```python
from build123d import *

# Parameters (mm, degrees)
SKETCH11_RX                  = 55.88
SKETCH11_RY                  = 50.8
BOSS_EXTRUDE4_DEPTH          = 9.525
SKETCH14_R                   = 0.0001
CUT_EXTRUDE5_DEPTH           = 10.525
CUT_EXTRUDE4_DEPTH           = 10.525
LPATTERN1_COUNT              = 4
LPATTERN1_PITCH              = 3.5
LPATTERN1_COL_COUNT          = 4
LPATTERN1_COL_PITCH          = 3.5
MIRROR1_COPY_1_DEPTH         = 10.525
MIRROR1_COPY_2_DEPTH         = 10.525
MIRROR1_COPY_3_DEPTH         = 10.525
MIRROR1_COPY_4_DEPTH         = 10.525
MIRROR1_COPY_5_DEPTH         = 10.525
MIRROR1_COPY_6_DEPTH         = 10.525
F_1_8_0_125_DIAMETER_HOLE1_D = 3.175


with BuildPart() as part:
    # Sketch11 → Boss-Extrude4 (new body)
    with BuildSketch(Plane(origin=(0, 0, 0), x_dir=(1, 0, 0), z_dir=(0, 1, 0))):
        with Locations(Location((0, 0), (0, 0, 180))):
            Ellipse(SKETCH11_RX, SKETCH11_RY)
        with BuildLine():
            Line((-32.5125, 22.448135593), (32.5125, 22.448135593))
            ThreePointArc((32.5125, 22.448135593), (40.370224106, 19.193359699), (43.625, 11.335635593))
            Line((43.625, 11.335635593), (43.625, -11.335635593))
            ThreePointArc((43.625, -11.335635593), (40.370224106, -19.193359699), (32.5125, -22.448135593))
            Line((32.5125, -22.448135593), (-32.5125, -22.448135593))
            ThreePointArc((-32.5125, -22.448135593), (-40.370224106, -19.193359699), (-43.625, -11.335635593))
            Line((-43.625, -11.335635593), (-43.625, 11.335635593))
            ThreePointArc((-43.625, 11.335635593), (-40.370224106, 19.193359699), (-32.5125, 22.448135593))
        make_face(mode=Mode.SUBTRACT)
    extrude(amount=BOSS_EXTRUDE4_DEPTH)

    # Sketch14 → Cut-Extrude5 (cut, through all)
    with BuildSketch(Plane(origin=(0, 9.525, 0), x_dir=(1, 0, 0), z_dir=(0, 1, 0))):
        with Locations((-25.4, 28.798235593)):
            Circle(SKETCH14_R)
        with Locations((25.4, 28.798235593)):
            Circle(SKETCH14_R)
        with Locations((25.4, 38.323035593)):
            Circle(SKETCH14_R)
        with Locations((-25.4, 38.323035593)):
            Circle(SKETCH14_R)
        with BuildLine():
            Line((-25.4, 38.323135593), (-6.981368472, 38.323135593))
            ThreePointArc((-6.981368472, 38.323135593), (-5.858836457, 38.788103578), (-5.393868472, 39.910635593))
            Line((-5.393868472, 39.910635593), (-5.393868472, 41.815635593))
            ThreePointArc((-5.393868472, 41.815635593), (-4.928900487, 42.938167608), (-3.806368472, 43.403135593))
            Line((-3.806368472, 43.403135593), (3.806368472, 43.403135593))
            ThreePointArc((3.806368472, 43.403135593), (4.928900487, 42.938167608), (5.393868472, 41.815635593))
            Line((5.393868472, 41.815635593), (5.393868472, 39.910635593))
            ThreePointArc((5.393868472, 39.910635593), (5.858836457, 38.788103578), (6.981368472, 38.323135593))
            Line((6.981368472, 38.323135593), (25.4001, 38.323035593))
            Line((25.4001, 38.323035593), (25.4, 28.798135593))
            Line((25.4, 28.798135593), (-25.4001, 28.798235593))
            Line((-25.4001, 28.798235593), (-25.4, 38.323135593))
        make_face()
    cut_extrude5 = extrude(amount=-CUT_EXTRUDE5_DEPTH, mode=Mode.SUBTRACT)

    # Sketch12 → Cut-Extrude4 (cut, through all)
    with BuildSketch(Plane(origin=(0, 9.525, 0), x_dir=(1, 0, 0), z_dir=(0, 1, 0))):
        with BuildLine():
            Line((-43.625, 0.81), (-47.625, 0.81))
            ThreePointArc((-47.625, 0.81), (-48.435, 0), (-47.625, -0.81))
            Line((-47.625, -0.81), (-43.625, -0.81))
            Line((-43.625, -0.81), (-43.625, 0.81))
        make_face()
    cut_extrude4 = extrude(amount=-CUT_EXTRUDE4_DEPTH, mode=Mode.SUBTRACT)

    # LPattern1: Cut-Extrude4 ×4
    with Locations(*[(0, 0, -i * LPATTERN1_PITCH) for i in range(1, LPATTERN1_COUNT)]):
        add(cut_extrude4, mode=Mode.SUBTRACT)

    # LPattern1 col: Cut-Extrude4 ×4
    with Locations(*[(0, 0, i * LPATTERN1_COL_PITCH) for i in range(1, LPATTERN1_COL_COUNT)]):
        add(cut_extrude4, mode=Mode.SUBTRACT)

    # Mirror1: Cut-Extrude4 across plane
    add(cut_extrude4.mirror(Plane(origin=(0, 0, 0), x_dir=(0, 0, 1), z_dir=(1, 0, 0))), mode=Mode.SUBTRACT)

    # Mirror1 copy 1 sketch → Mirror1 copy 1 (cut, through all)
    with BuildSketch(Plane(origin=(0, 9.525, -3.5), x_dir=(-1, 0, 0), z_dir=(0, 1, 0))):
        with BuildLine():
            Line((-43.625, -0.81), (-47.625, -0.81))
            ThreePointArc((-47.625, -0.81), (-48.435, 0), (-47.625, 0.81))
            Line((-47.625, 0.81), (-43.625, 0.81))
            Line((-43.625, 0.81), (-43.625, -0.81))
        make_face()
    extrude(amount=-MIRROR1_COPY_1_DEPTH, mode=Mode.SUBTRACT)

    # Mirror1 copy 2 sketch → Mirror1 copy 2 (cut, through all)
    with BuildSketch(Plane(origin=(0, 9.525, -7), x_dir=(-1, 0, 0), z_dir=(0, 1, 0))):
        with BuildLine():
            Line((-43.625, -0.81), (-47.625, -0.81))
            ThreePointArc((-47.625, -0.81), (-48.435, 0), (-47.625, 0.81))
            Line((-47.625, 0.81), (-43.625, 0.81))
            Line((-43.625, 0.81), (-43.625, -0.81))
        make_face()
    extrude(amount=-MIRROR1_COPY_2_DEPTH, mode=Mode.SUBTRACT)

    # Mirror1 copy 3 sketch → Mirror1 copy 3 (cut, through all)
    with BuildSketch(Plane(origin=(0, 9.525, -10.5), x_dir=(-1, 0, 0), z_dir=(0, 1, 0))):
        with BuildLine():
            Line((-43.625, -0.81), (-47.625, -0.81))
            ThreePointArc((-47.625, -0.81), (-48.435, 0), (-47.625, 0.81))
            Line((-47.625, 0.81), (-43.625, 0.81))
            Line((-43.625, 0.81), (-43.625, -0.81))
        make_face()
    extrude(amount=-MIRROR1_COPY_3_DEPTH, mode=Mode.SUBTRACT)

    # Mirror1 copy 4 sketch → Mirror1 copy 4 (cut, through all)
    with BuildSketch(Plane(origin=(0, 9.525, 3.5), x_dir=(-1, 0, 0), z_dir=(0, 1, 0))):
        with BuildLine():
            Line((-43.625, -0.81), (-47.625, -0.81))
            ThreePointArc((-47.625, -0.81), (-48.435, 0), (-47.625, 0.81))
            Line((-47.625, 0.81), (-43.625, 0.81))
            Line((-43.625, 0.81), (-43.625, -0.81))
        make_face()
    extrude(amount=-MIRROR1_COPY_4_DEPTH, mode=Mode.SUBTRACT)

    # Mirror1 copy 5 sketch → Mirror1 copy 5 (cut, through all)
    with BuildSketch(Plane(origin=(0, 9.525, 7), x_dir=(-1, 0, 0), z_dir=(0, 1, 0))):
        with BuildLine():
            Line((-43.625, -0.81), (-47.625, -0.81))
            ThreePointArc((-47.625, -0.81), (-48.435, 0), (-47.625, 0.81))
            Line((-47.625, 0.81), (-43.625, 0.81))
            Line((-43.625, 0.81), (-43.625, -0.81))
        make_face()
    extrude(amount=-MIRROR1_COPY_5_DEPTH, mode=Mode.SUBTRACT)

    # Mirror1 copy 6 sketch → Mirror1 copy 6 (cut, through all)
    with BuildSketch(Plane(origin=(0, 9.525, 10.5), x_dir=(-1, 0, 0), z_dir=(0, 1, 0))):
        with BuildLine():
            Line((-43.625, -0.81), (-47.625, -0.81))
            ThreePointArc((-47.625, -0.81), (-48.435, 0), (-47.625, 0.81))
            Line((-47.625, 0.81), (-43.625, 0.81))
            Line((-43.625, 0.81), (-43.625, -0.81))
        make_face()
    extrude(amount=-MIRROR1_COPY_6_DEPTH, mode=Mode.SUBTRACT)

    # Mirror2: Cut-Extrude5 across plane
    add(cut_extrude5.mirror(Plane.XY), mode=Mode.SUBTRACT)

    # 1_8 _0.125_ Diameter Hole1 (through all)
    with Locations(Plane(origin=(0, 9.525, 0), x_dir=(1, 0, 0), z_dir=(0, 1, 0))):
        with Locations((-25.4001, 28.798235593), (-25.4001, 38.323035593), (25.4001, 38.323035593), (25.4, 28.798135593), (-25.4, -28.798135593), (-25.4001, -38.323035593), (25.4, -28.798135593), (25.4001, -38.323035593)):
            Hole(F_1_8_0_125_DIAMETER_HOLE1_D / 2)


solid = part.part
```
CAD build for the part. Positions are in the model's coordinates, mm. Round coordinates to 2 decimals unless told otherwise and drop trailing zeros.
Q1. Slice it at A-A (x = 0.5). State how many separate pieces and enclosed holes the cut face has, and give its area (3 significant figures).
Q2. Drop flat-ended pins along their axis: pin 1 (1.9 mm diameter, centred on y = 4, z = 32, fed in from -X); pin 2 (4.5 mm diameter, centred on x = 45, y = 3, fed in from -Z); pin 3 (1.5 mm diameter, centred on y = 3, z = 5.5, fed in from -X). Give the stop position or say it passes through.
Q3. Two-plate mould, pull along Z, no slides. Class faces 1 (the flat face through (-46, 5, -2.69)), 2 (the flat face through (1, 9.525, 23)), 3 (the flat face through (-16, 5, -38.323)): pulls with the +Z half, pulls with the -Z half, needs draft (parallel to the pull), parting line crosses it, or undercut.
Q4. Wall check: L1, parallel to Z at x = -0.5, y = 2.5; L2, parallel to Z at x = -3.5, y = 6.25; L3, parallel to X at y = 4.25, z = -14.5. Give the ranges that are in metal, low to high.
Results below:
1. separate pieces: 4
1. enclosed holes: 0
1. area: 262 mm2
2. pin 1: stops at x = -44.23
2. pin 2: stops at z = -32.71
2. pin 3: stops at x = -55.64
3. face 1: undercut
3. face 2: needs draft
3. face 3: undercut
4. L1: z = -50.8 to -43.4, -28.8 to -22.45, 22.45 to 28.8, 43.4 to 50.8
4. L2: z = -50.7 to -43.4, -28.8 to -22.45, 22.45 to 28.8, 43.4 to 50.7
4. L3: x = -53.56 to -43.16, 43.16 to 53.56
